Here's how the part is built. I have some questions about the finished solid (model axes, mm). A direction names the side the tool comes from. Coordinates: 2 decimals unless noted, no trailing zeros. Write each loop counter-clockwise with the first axis right and the second up, starting at its lowest first coordinate (ties: lowest second). Pieces come first, ordered by that corner, then holes. Notation, with made-up numbers: M 3,-24.75 L 17,-24.75 A26 ccw 17,-8.75 Z; hole C 47,-10 d8. An arc over 180 degrees is marked long. Write each question's results on one line, items separated by ' | '. Start each with the question number.
from build123d import *

# Parameters (mm, degrees)
BOSS_EXTRUDE1_DEPTH = 20.32
CUT_EXTRUDE1_REACH  = 8.35
SKETCH2_R           = 6.985
CUT_EXTRUDE2_REACH  = 8.35
SKETCH3_R           = 6.985


with BuildPart() as part:
    # Sketch1 → Boss-Extrude1 (new body, symmetric)
    with BuildSketch(Plane.XY):
        with BuildLine():
            Line((0, 1.27), (0, 46.99))
            Line((0, 46.99), (-6.35, 46.99))
            Line((-6.35, 46.99), (-6.35, 1.27))
            ThreePointArc((-6.35, 1.27), (-4.118153673, -4.118153673), (1.27, -6.35))
            Line((1.27, -6.35), (40.64, -6.35))
            Line((40.64, -6.35), (40.64, 0))
            Line((40.64, 0), (1.27, 0))
            ThreePointArc((1.27, 0), (0.371974388, 0.371974388), (0, 1.27))
        make_face()
    extrude(amount=BOSS_EXTRUDE1_DEPTH, both=True)

    # Sketch2 → Cut-Extrude1 (cut, up to next)
    with BuildSketch(Plane(origin=(0, 0, 0), x_dir=(0, 0, -1), z_dir=(1, 0, 0)), mode=Mode.PRIVATE) as cut_extrude1_sk1:
        with Locations((0, 26.035)):
            Circle(SKETCH2_R)
    cut_extrude1_tool1 = extrude(cut_extrude1_sk1.sketch, amount=-CUT_EXTRUDE1_REACH, mode=Mode.PRIVATE) & part.part
    add(cut_extrude1_tool1.solids().sort_by_distance((0, 26.035, 0))[0], mode=Mode.SUBTRACT)

    # Sketch3 → Cut-Extrude2 (cut, up to next)
    with BuildSketch(Plane(origin=(0, 0, 0), x_dir=(1, 0, 0), z_dir=(0, 1, 0)), mode=Mode.PRIVATE) as cut_extrude2_sk1:
        with Locations((19.685, 0)):
            Circle(SKETCH3_R)
    cut_extrude2_tool1 = extrude(cut_extrude2_sk1.sketch, amount=-CUT_EXTRUDE2_REACH, mode=Mode.PRIVATE) & part.part
    add(cut_extrude2_tool1.solids().sort_by_distance((19.685, 0, 0))[0], mode=Mode.SUBTRACT)


solid = part.part
1) For pin 1 Ø4 at (x, z) = (34, -7.5) entering from +Y; pin 2 Ø10 at (y, z) = (19, 0.5) entering from +X, each with a flat end and sliding along its axis, tell me the tip position at first contact or that it passes through.
2) For faces 1 (the flat face through (-3, 46.99, 0)), 2 (the flat face through (0, 18.7, 0.3)), which set-ups out of +Z, -Z, +X, -X, +Y, -Y let a thin tool reach every point of the face, with its end or its side?
3) I want a section at D-D, the plane z = 13. Write out the boundary of the cut face in (x, y).
4) I want a section at B-B, the plane y = 21.5. Write out the boundary of the cut face in (x, z).
5) I want a section at C-C, the plane x = 19. Write out the boundary of the cut face in (y, z).
6) I want a section at A-A, the plane z = 0. Write out the boundary of the cut face in (x, y).
7) We'd pull the mould along Z, two halves only. Please class faces 3 (the flat face through (-0.4, 12.5, 20.32)), 4 (the flat face through (-0.4, 12.5, -20.32)), 5 (the cylindrical face through (-3.13, 32.96, 0.91)), 6 (the flat face through (-6.35, 19, 5)): pulls with the +Z half, pulls with the -Z half, needs draft (parallel to the pull), parting line crosses it, or undercut.
8) Please list where these lines run through material, in increasing order: line 1 (X direction, y = 4, z = 2.5); line 2 (Z direction, x = 19.5, y = -3.5). Write a range as [from, to].
Output:
1) pin 1: stops at y = 0 | pin 2: stops at x = 0
2) face 1: +Z, -Z, +X, -X, +Y | face 2: +Z, -Z, +X, +Y
3) outline: M -6.35,1.27 A7.62 ccw 1.27,-6.35 L 40.64,-6.35 L 40.64,0 L 1.27,0 A1.27 cw 0,1.27 L 0,46.99 L -6.35,46.99 Z
4) outline: M -6.35,-20.32 L 0,-20.32 L 0,-5.31 L -6.35,-5.31 Z; M -6.35,5.31 L 0,5.31 L 0,20.32 L -6.35,20.32 Z
5) outline: M -6.35,-20.32 L 0,-20.32 L 0,-6.95 L -6.35,-6.95 Z; M -6.35,6.95 L 0,6.95 L 0,20.32 L -6.35,20.32 Z
6) outline: M -6.35,1.27 A7.62 ccw 1.27,-6.35 L 12.7,-6.35 L 12.7,0 L 1.27,0 A1.27 cw 0,1.27 L 0,19.05 L -6.35,19.05 Z; M -6.35,33.02 L 0,33.02 L 0,46.99 L -6.35,46.99 Z; M 26.67,-6.35 L 40.64,-6.35 L 40.64,0 L 26.67,0 Z
7) face 3: pulls with the +Z half | face 4: pulls with the -Z half | face 5: undercut | face 6: needs draft
8) line 1: x = [-6.35, 0] | line 2: z = [-20.32, -6.98], [6.98, 20.32]
